Read the model definition and answer for the solid it produces. Units are mm, in the model's axes. A direction names the side the tool comes from. Coordinates: 2 decimals unless noted, no trailing zeros. Loops run counter-clockwise (first coordinate to the right, second up) from the corner with the lowest first, then second, coordinate; pieces in that order, holes last. Notation, with made-up numbers: M 41,-19 L 57,-19 A33 ccw 57,11 Z; hole C 35,19.5 d11. An arc over 180 degrees is marked long. One line per item, written item: value. Start each with the question number.
1. Consider probe 1 along Y at (x, z) = (-50, 5.75); probe 2 along X at (y, z) = (1.5, 4); probe 3 along Y at (x, z) = (9, 4.5). Determine where each line is inside the solid, lowest interval first.
2. The part is cut by section B-B (y = 0). Write down the section's boundary in (x, z) (3 decimals).
3. The part is cut by section C-C (z = 6.5). Write down the section's boundary in (x, y).
4. For faces 4 (the face through (-26.17, 13.336, 3.944)), 5 (the face through (-55, 18, 4)), 6 (the face through (-47, 14, 4)), determine the directions among +Z, -Z, +X, -X, +Y, -Y from which every point of the face is accessible in a straight line to the end or side of a thin tool.
5. The part is cut by section A-A (x = 50). Write down the section's boundary in (y, z) (3 decimals).
6. Determine the mould class of faces 1 (the face through (54, 21, 4)), 2 (the face through (0, -4, 4)), 3 (the face through (25.856, 13.089, 3.944)) for opening direction X: +X half, -X half, draft (parallel to the pull), parting line (faces both ways), or undercut.
7. The part is cut by section D-D (y = 11). Write down the section's boundary in (x, z), then the cut area to 3 significant figures.
8. Flat-ended cylindrical pins translate along their axes: pin 1 (1.5 mm diameter, centred on x = -19, z = 2.5, fed in from +Y); pin 2 (2.5 mm diameter, centred on x = -6, z = 2.5, fed in from +Y); pin 3 (8 mm diameter, centred on x = -32.5, y = 6.5, fed in from -Z); pin 4 (2 mm diameter, centred on y = 2, z = 6, fed in from +X). Find the tip coordinate at first contact, or state that the pin passes through.
```python
from build123d import *

# Parameters (mm, degrees)
SKETCH1_R                             = 1
BOSS_EXTRUDE1_DEPTH                   = 8
TAP_DRILL_FOR_M3X0_5_TAP1_D           = 2.5
TAP_DRILL_FOR_M3X0_5_TAP1_CSINK_D     = 2.55
TAP_DRILL_FOR_M3X0_5_TAP1_CSINK_ANGLE = 90
M3_CLEARANCE_HOLE1_D                  = 3.6
M3_CLEARANCE_HOLE1_CSINK_D            = 3.65
M3_CLEARANCE_HOLE1_CSINK_ANGLE        = 90
CHAMFER3_SIZE                         = 2
FILLET1_R                             = 2


with BuildPart() as part:
    # Sketch1 → Boss-Extrude1 (new body)
    with BuildSketch(Plane.XY):
        Polygon((-14.241705008, 4), (14.241705008, 4), (37.241705008, 22), (55, 22), (55, 14), (40, 14), (17, -4), (-17, -4), (-40, 14), (-55, 14), (-55, 22), (-37.241705008, 22), align=None)
        with Locations((16, 0)):
            Circle(SKETCH1_R, mode=Mode.SUBTRACT)
        with Locations((50, 18)):
            Circle(SKETCH1_R, mode=Mode.SUBTRACT)
        with Locations(Location((-50, 18, 0), (0, 0, 180))):
            Circle(SKETCH1_R, mode=Mode.SUBTRACT)
        with Locations(Location((-16, 0, 0), (0, 0, 180))):
            Circle(SKETCH1_R, mode=Mode.SUBTRACT)
    extrude(amount=BOSS_EXTRUDE1_DEPTH)

    # Tap Drill for M3x0.5 Tap1 (through all)
    with Locations(Plane.XY.offset(8)):
        with Locations((50, 18), (-50, 18)):
            CounterSinkHole(TAP_DRILL_FOR_M3X0_5_TAP1_D / 2, TAP_DRILL_FOR_M3X0_5_TAP1_CSINK_D / 2, counter_sink_angle=TAP_DRILL_FOR_M3X0_5_TAP1_CSINK_ANGLE)

    # M3 Clearance Hole1 (through all)
    with Locations(Plane.XY.offset(8)):
        with Locations((-16, 0), (16, 0)):
            CounterSinkHole(M3_CLEARANCE_HOLE1_D / 2, M3_CLEARANCE_HOLE1_CSINK_D / 2, counter_sink_angle=M3_CLEARANCE_HOLE1_CSINK_ANGLE)

    # Chamfer3
    chamfer3_edges = [part.edges().sort_by_distance(p)[0] for p in [
        (55, 22, 4),
        (55, 14, 4),
        (-55, 14, 4),
        (-55, 22, 4),
    ]]
    chamfer(chamfer3_edges, length=CHAMFER3_SIZE)

    # Fillet1
    fillet1_edges = [part.edges().sort_by_distance(p)[0] for p in [
        (40, 14, 4),
        (-40, 14, 4),
        (-14.241705008, 4, 4),
        (14.241705008, 4, 4),
    ]]
    fillet(fillet1_edges, radius=FILLET1_R)


solid = part.part
```
Answer block:
1. probe 1: y = 14 to 16.75, 19.25 to 22
1. probe 2: x = -24.03 to -16.99, -15.01 to 15.01, 16.99 to 24.03
1. probe 3: y = -4 to 4
2. outline: M -22.111,0 L -17.8,0 L -17.8,7.975 L -17.825,8 L -22.111,8 Z; M -14.2,0 L 14.2,0 L 14.2,7.975 L 14.175,8 L -14.175,8 L -14.2,7.975 Z; M 17.8,0 L 22.111,0 L 22.111,8 L 17.825,8 L 17.8,7.975 Z
3. outline: M -55,16 L -53,14 L -40.69,14 A2 cw -39.46,13.58 L -17,-4 L 17,-4 L 39.46,13.58 A2 cw 40.69,14 L 53,14 L 55,16 L 55,20 L 53,22 L 37.24,22 L 14.78,4.42 A2 cw 13.55,4 L -13.55,4 A2 cw -14.78,4.42 L -37.24,22 L -53,22 L -55,20 Z; hole C -50,18 d2.5; hole C -16,0 d3.6; hole C 16,0 d3.6; hole C 50,18 d2.5
4. face 4: +Z, -Z, +Y
4. face 5: +Z, -Z, -X, +Y, -Y
4. face 6: +Z, -Z, -X, -Y
5. outline: M 14,0 L 16.75,0 L 16.75,7.975 L 16.725,8 L 14,8 Z; M 19.25,0 L 22,0 L 22,8 L 19.275,8 L 19.25,7.975 Z
6. face 1: +X half
6. face 2: draft
6. face 3: undercut
7. outline: M -36.17,0 L -23.19,0 L -23.19,8 L -36.17,8 Z; M 23.19,0 L 36.17,0 L 36.17,8 L 23.19,8 Z
7. area: 208 mm2
8. pin 1: stops at y = 8.31
8. pin 2: stops at y = 4
8. pin 3: stops at z = 0
8. pin 4: stops at x = 25.94
